Design review of the part shown in the three views and the two pictorial views. Dimensions are in mm from the part's minimum x, y and z. Give positions to 0.01 mm unless a question says otherwise; leave off trailing zeros. Loops run counter-clockwise (first coordinate to the right, second up) from the corner with the lowest first, then second, coordinate; pieces in that order, holes last.
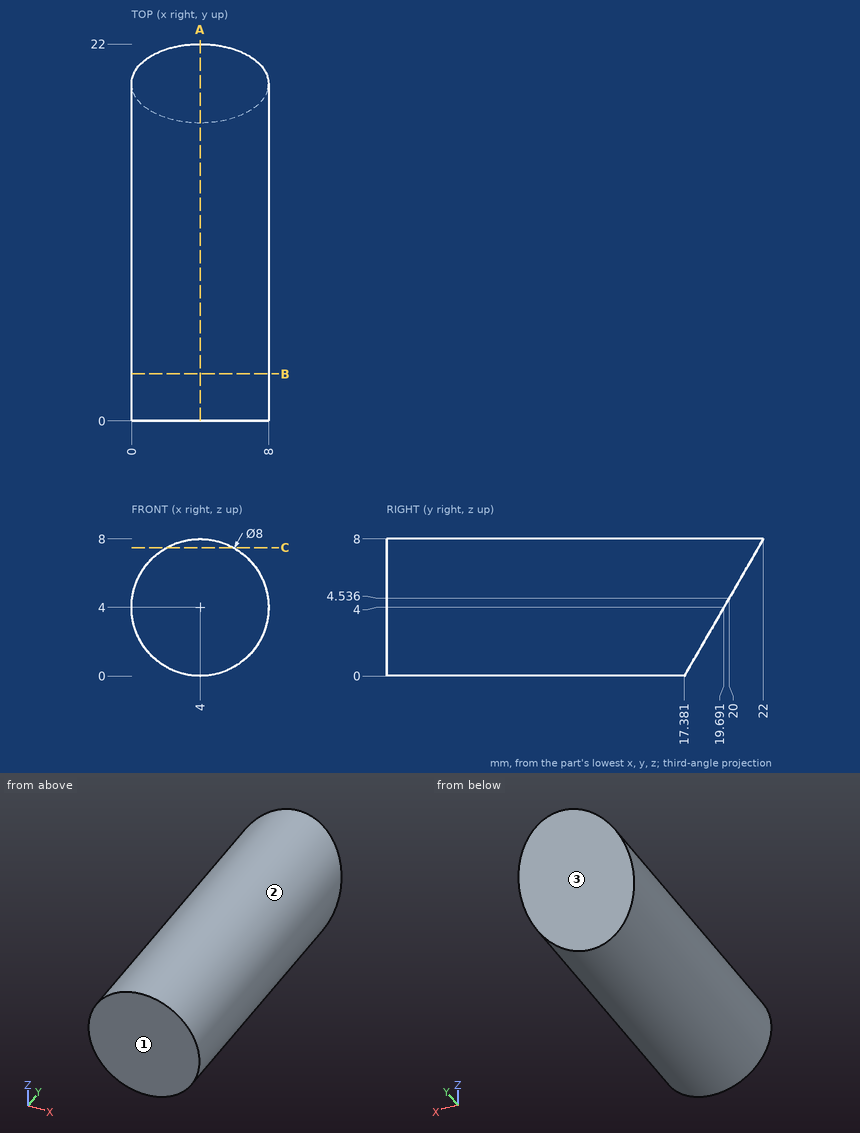
Q1. Take a section at C-C (z = 7.5). Give the boundary of the cut face in (x, y).
Results:
outline: (2.06, 0) - (5.94, 0) - (5.94, 21.71) - (2.06, 21.71) - close
Q2. Insertion check: pin 1 (1.5 mm diameter, centred on x = 2.5, y = 9.5, fed in from +Z); pin 2 (1 mm diameter, centred on y = 12.5, z = 4.5, fed in from +X); pin 3 (2 mm diameter, centred on y = 19.5, z = 2, fed in from -X) (1 decimal); pin 4 (1.5 mm diameter, centred on y = 10, z = 1, fed in from -X). Each pin has a flat end and moves straight along its axis. Give the tip position at first contact, or say it passes through.
Results:
pin 1: stops at z = 7.93
pin 2: stops at x = 8
pin 3: stops at x = 0.2
pin 4: stops at x = 0.69
Q3. Draft analysis for pull direction Z (two halves, no side actions). For the marked faces 1, 2 and 3, state which applies: pulls with the +Z half, pulls with the -Z half, needs draft (parallel to the pull), parting line crosses it, or undercut.
Results:
face 1: needs draft
face 2: parting line crosses it
face 3: pulls with the -Z half
Q4. Take a section at B-B (y = 2.75). Give the boundary of the cut face in (x, z).
Results:
outline: circle Ø8 at (4, 4)
Q5. Wall thickness on line 1 (Z direction, x = 1, y = 3) (1 decimal); line 2 (Y direction, x = 6.25, z = 5.5) (1 decimal); line 3 (Y direction, x = 1.5, z = 2.5) (1 decimal): over which ranges is each line inside the solid? List them lowest first.
Results:
line 1: z = 1.4 to 6.6
line 2: y = 0 to 20.6
line 3: y = 0 to 18.8
Q6. Take a section at A-A (x = 4). Give the boundary of the cut face in (y, z).
Results:
outline: (0, 0) - (17.38, 0) - (22, 8) - (0, 8) - close
